Input: dimensioned drawing with shaded views. Units: mm. Origin: part minimum x, y, z. Round coordinates to 2 decimals unless told otherwise and drop trailing zeros. Write each loop counter-clockwise with the first axis right and the second up, starting at its lowest first coordinate (ties: lowest second). Pieces come first, ordered by that corner, then holes. Notation, with made-up numbers: M 30,55 L 72,55 A22 ccw 72,71 Z; hole C 55,-9.75 d8. An arc over 180 degrees is marked long. Answer in a Markdown table with one row per item. Add a question column.
Item 1: Contact query for flat-ended pins moving along their axis: pin 1 (2.5 mm diameter, centred on y = 56, z = 1.5, fed in from +X); pin 2 (3 mm diameter, centred on x = 95.5, z = 2.5, fed in from -Y); pin 3 (1.5 mm diameter, centred on y = 176.5, z = 2.5, fed in from -X). Output: stop coordinate, or through.
Item 2: Material intervals for probe 1 along X at (y, z) = (54, 3.55), sorted ascending.
Item 3: Cut plane A-A on y = 100. Return loops of the section in (x, z).
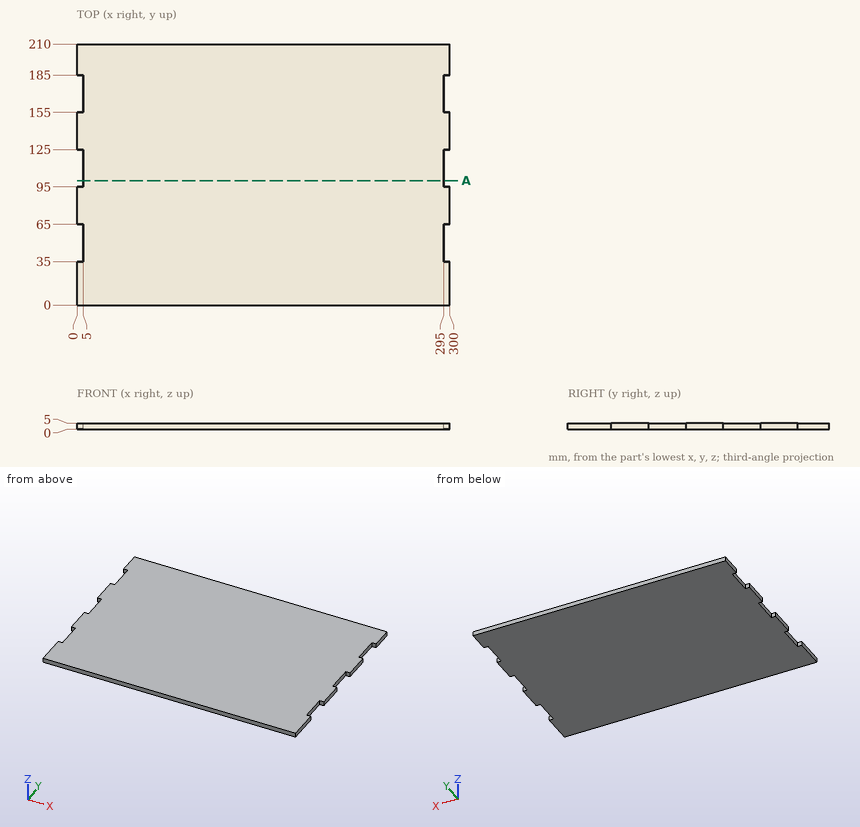
Results below:
| question | item | result |
|---|---|---|
| 1 | pin 1 | x = 295 |
| 1 | pin 2 | y = 0 |
| 1 | pin 3 | x = 5 |
| 2 | probe 1 | 5 to 295 |
| 3 | outline | M 5,0 L 295,0 L 295,5 L 5,5 Z |
